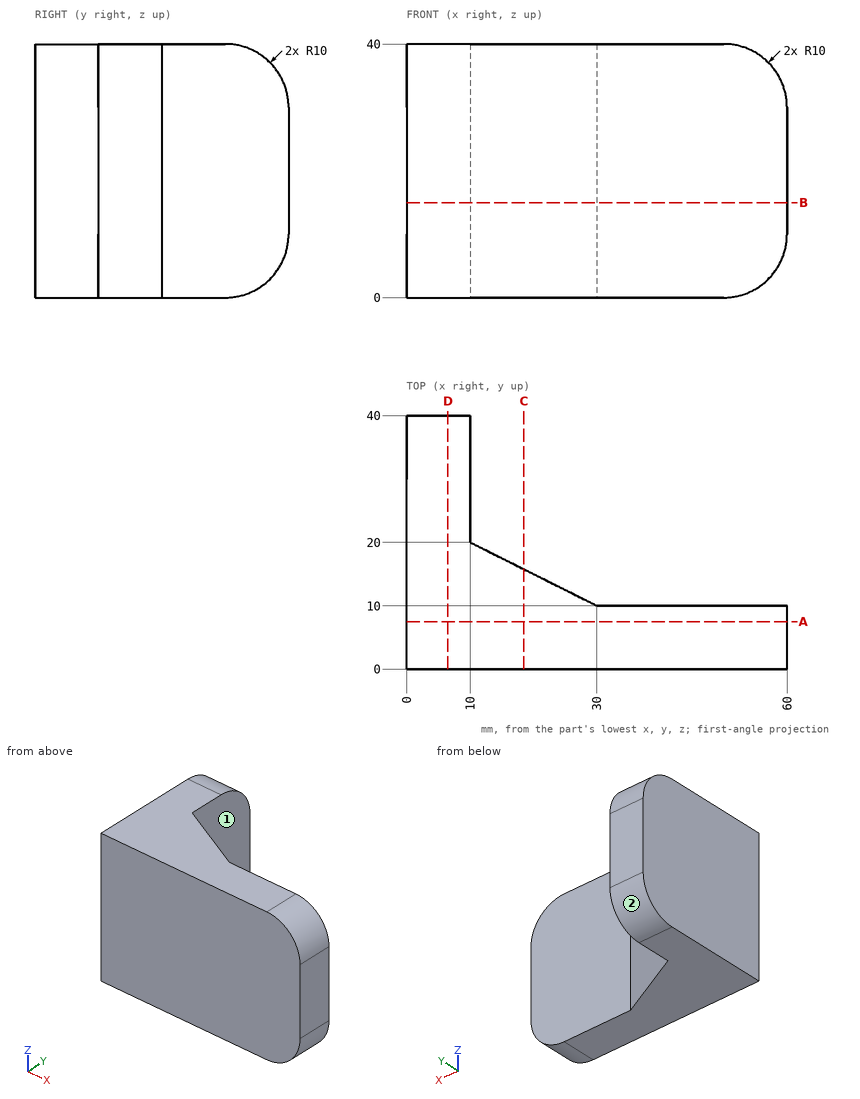
The figure shows three views and two pictorial views of one solid part (mm, origin at its lowest corner). Answer the questions. A direction names the side the tool comes from. Coordinates: 2 decimals unless noted, no trailing zeros. Loops run counter-clockwise (first coordinate to the right, second up) from the corner with the lowest first, then second, coordinate; pieces in that order, holes last. Notation, with made-up numbers: (-37, -2) -> (12, -2) arc R6 cw to (12, 9) -> close; hole circle Ø7 at (52.5, 65). An arc over 180 degrees is marked (long way). Use one line per item in the form item = value. Start each with the question number.
Item 1: Flat-ended cylindrical pins translate along their axes: pin 1 Ø12 at (x, z) = (39.5, 14) entering from +Y; pin 2 Ø16 at (y, z) = (27, 26) entering from +X; pin 3 Ø3 at (x, y) = (36.5, 10.5) entering from +Z; pin 4 Ø3 at (y, z) = (23, 21) entering from +X. Find the tip coordinate at first contact, or state that the pin passes through.
Item 2: The part is cut by section B-B on z = 15. Determine the outline of the cut face in (x, y), then the cut area to 3 significant figures.
Item 3: The part is cut by section C-C on x = 18.5. Determine the outline of the cut face in (y, z), then the cut area to 3 significant figures.
Item 4: A tool of negligible diameter and unlimited length cuts with its end or side. For the marked faces 1 and 2, from which of +Z, -Z, +X, -X, +Y, -Y can it reach the whole face along a straight path? Write none if from no direction.
Item 5: The part is cut by section A-A on y = 7.5. Determine the outline of the cut face in (x, z), then the cut area to 3 significant figures.
Item 6: Consider L1, parallel to Y at x = 41, z = 9.5; L2, parallel to Y at x = 7, z = 34.5. Determine where each line is inside the solid, lowest interval first. Write a range as [from, to].
Item 7: The part is cut by section D-D on x = 6.5. Determine the outline of the cut face in (y, z).
Answer key:
q1.pin_1 = 10
q1.pin_2 = 12
q1.pin_3 = 40
q1.pin_4 = 10
q2.outline = (0, 0) -> (60, 0) -> (60, 10) -> (30, 10) -> (10, 20) -> (10, 40) -> (0, 40) -> close
q2.area = 1,000 mm2
q3.outline = (0, 0) -> (15.75, 0) -> (15.75, 40) -> (0, 40) -> close
q3.area = 630 mm2
q4.face_1 = +Z, -Z, +X, +Y
q4.face_2 = -Z, +X, -X, +Y
q5.outline = (0, 0) -> (50, 0) arc R10 ccw to (60, 10) -> (60, 30) arc R10 ccw to (50, 40) -> (0, 40) -> close
q5.area = 2,360 mm2
q6.L1 = [0, 10]
q6.L2 = [0, 38.93]
q7.outline = (0, 0) -> (30, 0) arc R10 ccw to (40, 10) -> (40, 30) arc R10 ccw to (30, 40) -> (0, 40) -> close
